from build123d import *

# Parameters (mm, degrees)
ARM1_DEPTH          = 10
SKETCH3_R           = 15
BOSS_EXTRUDE2_DEPTH = 10


with BuildPart() as part:
    # Sketch1 → arm1 (new body)
    with BuildSketch(Plane(origin=(0, 0, 0), x_dir=(1, 0, 0), z_dir=(0, 1, 0))):
        with BuildLine():
            Line((-45, 10), (45, 10))
            ThreePointArc((45, 10), (55, 0), (45, -10))
            Line((45, -10), (-45, -10))
            Line((-45, -10), (-45, 10))
        make_face()
    extrude(amount=ARM1_DEPTH)

    # Sketch3 → Boss-Extrude2 (add)
    with BuildSketch(Plane(origin=(0, 10, 0), x_dir=(1, 0, 0), z_dir=(0, 1, 0))):
        with Locations(Location((45, 0, 0), (0, 0, 138.189685104))):
            Circle(SKETCH3_R)
    extrude(amount=BOSS_EXTRUDE2_DEPTH)


solid = part.part
Work out the finished part from the listing and answer in its coordinate system (mm). A direction names the side the tool comes from. Give positions to 0.01 mm unless a question says otherwise; leave off trailing zeros. Loops run counter-clockwise (first coordinate to the right, second up) from the corner with the lowest first, then second, coordinate; pieces in that order, holes last. Notation, with made-up numbers: (21.5, 0) -> (49.5, 0) arc R36 cw to (49.5, 36) -> close; hole circle Ø2 at (9.25, 24.5). An arc over 180 degrees is marked (long way). Use a Markdown table: item, result. Add a question column.
1. Section B-B on x = 44 is taken. Determine the outline of the cut face in (y, z).
2. Section C-C on y = 4 is taken. Determine the outline of the cut face in (x, z).
3. Find the intervals of material crossed by probe 1 along Y at (x, z) = (56.5, 1); probe 2 along Z at (x, y) = (-34.5, 3.75); probe 3 along Y at (x, z) = (9.5, 5.25), in increasing order.
4. Section A-A on z = 0 is taken. Determine the outline of the cut face in (x, y).
5. Flat-ended cylindrical pins translate along their axes: pin 1 Ø1 at (x, y) = (-29.5, 6) entering from +Z; pin 2 Ø10 at (x, z) = (6, -10.5) entering from +Y; pin 3 Ø12 at (y, z) = (2.5, 1.5) entering from +X. Find the tip coordinate at first contact, or state that the pin passes through.
6. Section D-D on x = 23 is taken. Determine the outline of the cut face in (y, z), and give its area (3 significant figures).
7. For faces 1 (the cylindrical face through (38.5, 14.93, -13.52)), 2 (the flat face through (56, 10, 1)), 3 (the flat face through (45, 20, 0)), determine the directions among +Z, -Z, +X, -X, +Y, -Y from which every point of the face is accessible in a straight line to the end or side of a thin tool.
Results below:
| question | item | result |
|---|---|---|
| 1 | outline | (0, -10) -> (10, -10) -> (10, -14.97) -> (20, -14.97) -> (20, 14.97) -> (10, 14.97) -> (10, 10) -> (0, 10) -> close |
| 2 | outline | (-45, -10) -> (45, -10) arc R10 ccw to (45, 10) -> (-45, 10) -> close |
| 3 | probe 1 | y = 10 to 20 |
| 3 | probe 2 | z = -10 to 10 |
| 3 | probe 3 | y = 0 to 10 |
| 4 | outline | (-45, 0) -> (55, 0) -> (55, 10) -> (60, 10) -> (60, 20) -> (30, 20) -> (30, 10) -> (-45, 10) -> close |
| 5 | pin 1 | stops at z = 10 |
| 5 | pin 2 | stops at y = 10 |
| 5 | pin 3 | stops at x = 55 |
| 6 | outline | (0, -10) -> (10, -10) -> (10, 10) -> (0, 10) -> close |
| 6 | area | 200 mm^2 |
| 7 | face 1 | +Y |
| 7 | face 2 | +X, -Y |
| 7 | face 3 | +Z, -Z, +X, -X, +Y |
